The listing builds one solid part. Answer for the finished solid, in the listing's coordinates (mm). Give positions to 0.01 mm unless a question says otherwise; leave off trailing zeros. Loops run counter-clockwise (first coordinate to the right, second up) from the corner with the lowest first, then second, coordinate; pieces in that order, holes last. Notation, with made-up numbers: M 43.5,38 L 57.5,38 A21 cw 57.5,45 Z; hole C -38,-6.5 d11. An arc over 180 degrees is marked long. Return JSON: item names as keys, results as strings.
from build123d import *

# Parameters (mm, degrees)
F0_W     = 914.4
F0_H     = 88.9
F1_DEPTH = 38.1
F2_W     = 152.4
F2_H     = 25.4
F3_DEPTH = 6.35
F4_R     = 6.35
F5_DEPTH = 25.4


with BuildPart() as f1:
    # F0 (on Top) → F1 (new body)
    with BuildSketch(Plane.XY):
        with Locations((-483.326185, -13.443414)):
            Rectangle(F0_W, F0_H)
    extrude(amount=F1_DEPTH)

    # F2 (on face) → F3 (join)
    with BuildSketch(Plane(origin=(0, 31.006586, 0), x_dir=(-1, 0, 0), z_dir=(0, 1, 0))):
        with Locations((127.726185, 19.05)):
            Rectangle(F2_W, F2_H)
    extrude(amount=F3_DEPTH)

    # F4 (on face) → F5 (cut)
    with BuildSketch(Plane(origin=(0, 31.006586, 0), x_dir=(-1, 0, 0), z_dir=(0, 1, 0))):
        with Locations((800.826185, 19.05)):
            Circle(F4_R)
    extrude(amount=-F5_DEPTH, mode=Mode.SUBTRACT)


solid = f1.part
(1) Given pin 1 (3 mm diameter, centred on x = -131.5, y = 35, fed in from +Z); pin 2 (3 mm diameter, centred on x = -161.5, y = 33.5, fed in from -Z); pin 3 (20.5 mm diameter, centred on x = -800.83, z = 19.05, fed in from +Y), each flat-ended and moving along its own axis, determine where each tip first touches the part or whether it passes through.
Values follow:
{"pin 1": "z = 31.75", "pin 2": "z = 6.35", "pin 3": "y = 31.01"}
(2) Straight lines are drawn through the part: line 1 along X through (y, z) = (12, 19); line 2 along Y through (x, z) = (-606.5, 10); line 3 along X through (y, z) = (13.5, 22). For each, find the intervals that lie inside material, in ascending order.
Values follow:
{"line 1": "-940.53 to -807.18, -794.48 to -26.13", "line 2": "-57.89 to 31.01", "line 3": "-940.53 to -806.45, -795.2 to -26.13"}
(3) The part is cut by section A-A (z = 19.05). Determine the outline of the cut face in (x, y).
Values follow:
{"outline": "M -940.53,-57.89 L -26.13,-57.89 L -26.13,31.01 L -51.53,31.01 L -51.53,37.36 L -203.93,37.36 L -203.93,31.01 L -794.48,31.01 L -794.48,5.61 L -807.18,5.61 L -807.18,31.01 L -940.53,31.01 Z"}
